Geometry check sheet. Reference: the model listing, model coordinates, mm. A direction names the side the tool comes from. Give positions to 0.01 mm unless a question says otherwise; leave off trailing zeros. Order: outer loops, then holes, each group sorted by start corner. A loop starts at its lowest first (then second) coordinate and runs counter-clockwise, first axis right, second up. Notation, with made-up numbers: M -27.75,86 L -13.75,86 A33 ccw -13.75,119 Z; hole C -28.5,47 d5. An arc over 180 degrees is marked long. Answer as CSV lines item,"result". Start each with the question number.
Q1. Section check A-A, the plane x = 55. Record the boundary of the cut face in (y, z) (3 decimals).
Q2. Thickness scan on line 1 (Y direction, x = -35, z = -0.25) (3 decimals); line 2 (Y direction, x = 19, z = 0.05) (3 decimals); line 3 (Y direction, x = 37, z = 0). Record the ranges inside material, lowest first.
Q3. Go/stop test with flat-tipped pins: pin 1 (2.5 mm diameter, centred on x = -10, y = -49, fed in from -Z); pin 2 (1.2 mm diameter, centred on y = -19, z = 0.5, fed in from +X); pin 3 (2 mm diameter, centred on y = -33.5, z = 0, fed in from +X); pin 4 (2 mm diameter, centred on x = -50, z = 0, fed in from +Y). Record where each tip stops, or that it passes through.
Q4. Section check B-B, the plane y = -14. Record the boundary of the cut face in (x, z), then the cut area to 3 significant figures.
Q5. Set-up check for faces 5 (the flat face through (25, -16, 0)), 6 (the flat face through (0, 0, 0)), 7 (the flat face through (-45, -33, 0)): record each of +Z, -Z, +X, -X, +Y, -Y from which the full face is reachable in a straight line by a thin tool's end or side.
Q6. Section check D-D, the plane x = -19. Record the boundary of the cut face in (y, z) (3 decimals).
Q7. Section check C-C, the plane z = -0.8. Count the separate pieces of the cut face and the enclosed holes in it, then the cut area to 3 significant figures.
Q8. Mould release check, pull along X, two halves, no side actions. Record for faces 1 (the cylindrical face through (-53.876, -47.969, -0.028)), 2 (the cylindrical face through (-33.476, -48.933, -0.028)), 3 (the cylindrical face through (-25.9, -32.14, 0.03)), 4 (the flat face through (1, -32, 2)): +X half, -X half, draft (parallel to the pull), parting line (faces both ways), or undercut.
```python
from build123d import *

# Parameters (mm, degrees)
EXTRUDE_1_DEPTH          = 2
FILLET_1_R               = 3
SKETCH_2_R               = 2.025
CUT_EXTRUDE_1_DEPTH      = 1
CUT_EXTRUDE_1_DEPTH_BACK = 5
SKETCH_3_R               = 1.525
CUT_EXTRUDE_2_DEPTH      = 10
SKETCH_4_R               = 10.5
CUT_EXTRUDE_3_DEPTH      = 5


with BuildPart() as part:
    # 草图1 → 凸台-拉伸1 (new body, symmetric)
    with BuildSketch(Plane.XY):
        Polygon((-25, 0), (25, 0), (25, -33), (65, -33), (65, -53), (-65, -53), (-65, -33), (-25, -33), align=None)
    extrude(amount=EXTRUDE_1_DEPTH, both=True)

    # 圆角1
    fillet_1_edges = [part.edges().sort_by_distance(p)[0] for p in [
        (-25, 0, 0),
        (25, 0, 0),
        (25, -33, 0),
        (65, -33, 0),
        (65, -53, 0),
        (-65, -53, 0),
        (-65, -33, 0),
        (-25, -33, 0),
    ]]
    fillet(fillet_1_edges, radius=FILLET_1_R)

    # 草图2 → 切除-拉伸1 (cut, two sides)
    with BuildSketch(Plane.XY.offset(2)) as cut_extrude_1_sk:
        with Locations((-19, -5)):
            Circle(SKETCH_2_R)
        with Locations((-19, -23)):
            Circle(SKETCH_2_R)
        with Locations((19, -5)):
            Circle(SKETCH_2_R)
        with Locations((19, -23)):
            Circle(SKETCH_2_R)
    extrude(amount=CUT_EXTRUDE_1_DEPTH, mode=Mode.SUBTRACT)
    extrude(cut_extrude_1_sk.sketch, amount=-CUT_EXTRUDE_1_DEPTH_BACK, mode=Mode.SUBTRACT)

    # 草图3 → 切除-拉伸2 (cut)
    with BuildSketch(Plane(origin=(0, 0, -2), x_dir=(-1, 0, 0), z_dir=(0, 0, -1))):
        with Locations((-55, -49)):
            Circle(SKETCH_3_R)
        with Locations((-35, -49)):
            Circle(SKETCH_3_R)
        with Locations((-10, -49)):
            Circle(SKETCH_3_R)
        with Locations((10, -49)):
            Circle(SKETCH_3_R)
        with Locations((35, -49)):
            Circle(SKETCH_3_R)
        with Locations((55, -49)):
            Circle(SKETCH_3_R)
        with Locations((55, -37)):
            Circle(SKETCH_3_R)
        with Locations((35, -37)):
            Circle(SKETCH_3_R)
        with Locations((10, -37)):
            Circle(SKETCH_3_R)
        with Locations((-10, -37)):
            Circle(SKETCH_3_R)
        with Locations((-35, -37)):
            Circle(SKETCH_3_R)
        with Locations((-55, -37)):
            Circle(SKETCH_3_R)
    extrude(amount=-CUT_EXTRUDE_2_DEPTH, mode=Mode.SUBTRACT)

    # 草图4 → 切除-拉伸3 (cut, through all)
    with BuildSketch(Plane.XY.offset(2)):
        with Locations((0, -14)):
            Circle(SKETCH_4_R)
    extrude(amount=-CUT_EXTRUDE_3_DEPTH, mode=Mode.SUBTRACT)


solid = part.part
```
Answer block:
1,outline,"M -53,-2 L -50.525,-2 L -50.525,2 L -53,2 Z; M -47.475,-2 L -38.525,-2 L -38.525,2 L -47.475,2 Z; M -35.475,-2 L -33,-2 L -33,2 L -35.475,2 Z"
2,line 1,"y = -53 to -50.525, -47.475 to -38.525, -35.475 to -33"
2,line 2,"y = -53 to -25.025, -20.975 to -7.025, -2.975 to 0"
2,line 3,"y = -53 to -33"
3,pin 1,"passes through"
3,pin 2,"stops at x = 25"
3,pin 3,"stops at x = 64.6"
3,pin 4,"stops at y = -33"
4,outline,"M -25,-2 L -10.5,-2 L -10.5,2 L -25,2 Z; M 10.5,-2 L 25,-2 L 25,2 L 10.5,2 Z"
4,area,"116 mm2"
5,face 5,"+Z, -Z, +X, +Y"
5,face 6,"+Z, -Z, +X, -X, +Y"
5,face 7,"+Z, -Z, -X, +Y"
6,outline,"M -53,-2 L -25.025,-2 L -25.025,2 L -53,2 Z; M -20.975,-2 L -7.025,-2 L -7.025,2 L -20.975,2 Z; M -2.975,-2 L 0,-2 L 0,2 L -2.975,2 Z"
7,separate pieces,"1"
7,enclosed holes,"17"
7,area,"3,760 mm2"
8,face 1,"undercut"
8,face 2,"undercut"
8,face 3,"-X half"
8,face 4,"draft"
